Part model, mm, in its own coordinate system. A direction names the side the tool comes from. Round coordinates to 2 decimals unless told otherwise and drop trailing zeros. Write each loop counter-clockwise with the first axis right and the second up, starting at its lowest first coordinate (ties: lowest second). Pieces come first, ordered by that corner, then holes. Notation, with made-up numbers: M -5,66 L 23,66 A34 cw 23,98 Z; hole C 42,60 d1. An arc over 180 degrees is marked long. Use a Markdown table: item, result. Add a question column.
1) Wall check: probe 1 along Y at (x, z) = (0, 1.7); probe 2 along Z at (x, y) = (3.25, -3.25); probe 3 along Y at (x, z) = (6.25, -1.75). Give the ranges that are in metal, low to high.
2) Two-plate mould, pull along X, no slides. Class faces 4 (the face through (7, -2, -8)), 5 (the face through (3.2, 0.1, 0)), 6 (the face through (-1.94, 8.735, 1.085)), 7 (the face through (-10.177, 0.148, -4.056)): released by +X, released by -X, zero draft, split by the parting line, or undercut.
3) Which spindle directions (+Z, -Z, +X, -X, +Y, -Y) get a long thin tool onto all of the face, cutting with end or side? Do faces 1 (the face through (4.3, -8.1, 0)), 2 (the face through (-5.424, 3.303, -3.944)), 3 (the face through (-5, -8, 0)). Say none if no direction does.
4) Slice it at A-A on x = -2.5. Write the cut outline in (y, z).
5) Slice it at D-D on x = 2.25. Write the cut outline in (y, z), plus the area to 3 significant figures.
6) Slice it at B-B on z = -0.75. Write the cut outline in (x, y), plus the area to 3 significant figures.
7) Drop flat-ended pins along their axis: P1, Ø2, axis at x = 1.5, z = 0, coming from the -Y side; P2, Ø6, axis at y = 5, z = -5, coming from the +X side; P3, Ø1.2, axis at x = 9.5, y = 2, coming from the +Z side. Give the stop position or say it passes through.
8) Slice it at C-C on y = -7.25. Write the cut outline in (x, z).
Autodesk Inventor part; units mm, degrees
ref_plane "YZ Plane" through (0, 0, 0) normal (1, 0, 0) x (0, 1, 0)
ref_plane "XZ Plane" through (0, 0, 0) normal (0, 1, 0) x (-1, 0, 0)
ref_plane "XY Plane" through (0, 0, 0) normal (0, 0, 1) x (1, 0, 0)
sketch "Sketch2" plane through (0, 0, 0) normal (0, 0, 1) x (1, 0, 0)
  line L0 (3.7629, 6.2932) -> (-3.5686, 6.4054)
  line L1 (-3.5686, 6.4054) -> (-7.3315, 0.1122)
  line L2 (-7.3315, 0.1122) -> (-3.7629, -6.2932)
  line L3 (-3.7629, -6.2932) -> (3.5686, -6.4054)
  line L4 (3.5686, -6.4054) -> (7.3315, -0.1122)
  line L5 (7.3315, -0.1122) -> (3.7629, 6.2932)
  line L6 (3.5686, -6.4054) -> (-3.5686, 6.4054)
  line L7 (-3.5686, 6.4054) -> (-5.0286, 9.0261)
  line L8 (7.3315, -0.1122) -> (-7.3315, 0.1122)
  line L9 (-5.0286, 9.0261) -> (5.3025, 8.868)
  line L10 (5.3025, 8.868) -> (10.3311, -0.1581)
  line L11 (10.3311, -0.1581) -> (5.0286, -9.0261)
  line L12 (5.0286, -9.0261) -> (-5.3025, -8.868)
  line L13 (-5.3025, -8.868) -> (-10.3311, 0.1581)
  line L14 (-10.3311, 0.1581) -> (-5.0286, 9.0261)
  line L15 (-3.5686, 6.4054) -> (3.7629, 6.2932)
  line L16 (3.7629, 6.2932) -> (7.3315, -0.1122)
  line L17 (7.3315, -0.1122) -> (3.5686, -6.4054)
  line L18 (3.5686, -6.4054) -> (-3.7629, -6.2932)
  line L19 (-3.7629, -6.2932) -> (-7.3315, 0.1122)
  line L20 (-7.3315, 0.1122) -> (-3.5686, 6.4054)
  point P0 (0, 0)
  point P1 (0, 0)
  point P2 (0, 0)
  dimension "d0" = 3
extrude "Extrusion1" add sketch "Sketch2" against normal blind 8
sketch "Sketch3" plane through (0, 0, 0) normal (0, 0, 1) x (1, 0, 0)
  line L0 (-5.0286, 9.0261) -> (-10.3311, 0.1581)
  line L1 (-5.3025, -8.868) -> (5.0286, -9.0261)
  line L2 (10.3311, -0.1581) -> (5.3025, 8.868)
  circle A0 centre (0, 0) radius 8.9481
  circle A1 centre (0, 0) radius 3
  point P0 (0, 0)
  dimension "d3" = 6
extrude "Extrusion2" add sketch "Sketch3" along normal blind 2.2
fillet "Fillet1" radius 1 6 edges at (-5.3025, -8.868, -4) (-10.3311, 0.1581, -4) (-5.0286, 9.0261, -4) (5.3025, 8.868, -4) (10.3311, -0.1581, -4) (5.0286, -9.0261, -4)
properties part number "MagnetHolder 6mm"
Entries:
| question | item | result |
|---|---|---|
| 1 | probe 1 | y = -8.95 to -3, 3 to 8.95 |
| 1 | probe 2 | z = 0 to 2.2 |
| 1 | probe 3 | y = -6.98 to -1.92, 1.83 to 7.17 |
| 2 | face 4 | zero draft |
| 2 | face 5 | undercut |
| 2 | face 6 | split by the parting line |
| 2 | face 7 | released by -X |
| 3 | face 1 | +Z, +X, -Y |
| 3 | face 2 | -Z |
| 3 | face 3 | +Z, -X, -Y |
| 4 | outline | M -8.91,-8 L -6.31,-8 L -6.31,0 L -1.66,0 L -1.66,2.2 L -8.59,2.2 L -8.59,0 L -8.91,0 Z; M 1.66,0 L 6.39,0 L 6.39,-8 L 8.99,-8 L 8.99,0 L 8.59,0 L 8.59,2.2 L 1.66,2.2 Z |
| 5 | outline | M -8.98,-8 L -6.39,-8 L -6.39,0 L -1.98,0 L -1.98,2.2 L -8.66,2.2 L -8.66,0 L -8.98,0 Z; M 1.98,0 L 6.32,0 L 6.32,-8 L 8.91,-8 L 8.91,0 L 8.66,0 L 8.66,2.2 L 1.98,2.2 Z |
| 5 | area | 70.9 mm^2 |
| 6 | outline | M -10.05,-0.35 L -5.58,-8.36 A1 ccw -4.73,-8.88 L 4.45,-9.02 A1 ccw 5.32,-8.53 L 10.03,-0.65 A1 ccw 10.05,0.35 L 5.58,8.36 A1 ccw 4.73,8.88 L -4.45,9.02 A1 ccw -5.32,8.53 L -10.03,0.65 A1 ccw Z; hole M -7.33,0.11 L -3.76,-6.29 L 3.57,-6.41 L 7.33,-0.11 L 3.76,6.29 L -3.57,6.41 Z |
| 6 | area | 137 mm^2 |
| 7 | P1 | stops at y = -8.99 |
| 7 | P2 | stops at x = 9.13 |
| 7 | P3 | stops at z = 0 |
| 8 | outline | M -6.2,-8 L 6.09,-8 L 6.09,0 L 5.24,0 L 5.24,2.2 L -5.24,2.2 L -5.24,0 L -6.2,0 Z |
